The model under review builds one solid part; all positions refer to its coordinate system, in mm. Face numbers are marked on the shaded views. Round coordinates to 2 decimals unless told otherwise and drop trailing zeros. Order: outer loops, then holes, each group sorted by start corner. A loop starts at its lowest first (then second) coordinate and runs counter-clockwise, first axis right, second up. Notation, with made-up numbers: M 79.5,51 L 110.5,51 A9 cw 110.5,64 Z; hole C -25.5,-30 d9. An arc over 180 degrees is marked long. Answer as a JSON object with one key per item and string values. Group by question number.
1. Add section D-D on y = 40. State the section outline as (x, z) points, and give its area (4 significant figures).
2. To check wall thickness, follow probe 1 along X at (y, z) = (7.5, 1.4); probe 2 along X at (y, z) = (49.5, 0.75); probe 3 along Y at (x, z) = (-31, 3.5). State the ranges of each line that lie inside material, in increasing order. Write a range as [from, to].
3. Add section A-A on y = 61. State the section outline as (x, z) points, and give its area (3 significant figures).
4. Add section C-C on z = 1.65. Give the number of separate pieces and of enclosed holes in the cut face, and give its area (3 significant figures).
5. Clearance check with a flat-ended pin moving along its axis: P1, Ø1.5, axis at x = -38.5, y = 20.5, coming from the -Z side. State where the tip first meets the part, or that it passes through.
6. Add section B-B on x = -39.5. State the section outline as (y, z) points, and give its area (3 significant figures).
7. Mouldability with a two-part tool opening along Y and no side actions: class the marked faces 1, 2 and 3 as released by +Y, released by -Y, zero draft, split by the parting line, or undercut.
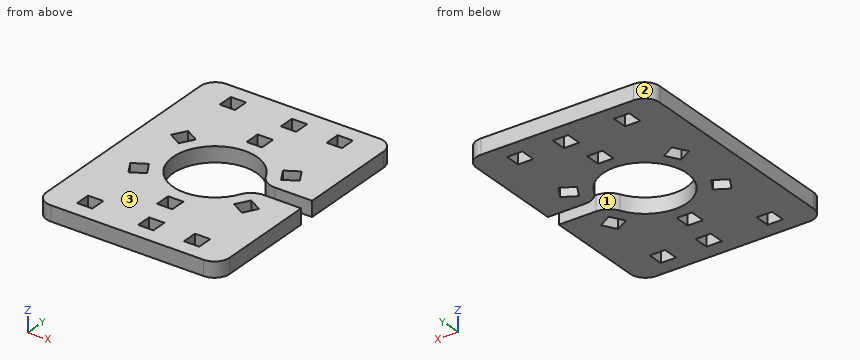
```python
from build123d import *

# Parameters (mm, degrees)
ESQUISSE1_W        = 5
ESQUISSE1_H        = 5
BOSS_EXTRU_1_DEPTH = 5


with BuildPart() as part:
    # Esquisse1 → Boss.-Extru.1 (new body)
    with BuildSketch(Plane.XY):
        with BuildLine():
            Line((-55, 80), (-5, 80))
            ThreePointArc((-5, 80), (-1.464466094, 78.535533906), (0, 75))
            Line((0, 75), (0, 42.5))
            Line((0, 42.5), (-12.172703514, 42.5))
            ThreePointArc((-12.172703514, 42.5), (-15.374759815, 43.42586604), (-17.588591054, 45.917721519))
            ThreePointArc((-17.588591054, 45.917721519), (-43.75, 40), (-17.588591054, 34.082278481))
            ThreePointArc((-17.588591054, 34.082278481), (-15.374759815, 36.57413396), (-12.172703514, 37.5))
            Line((-12.172703514, 37.5), (0, 37.5))
            Line((0, 37.5), (0, 5))
            ThreePointArc((0, 5), (-1.464466094, 1.464466094), (-5, 0))
            Line((-5, 0), (-55, 0))
            ThreePointArc((-55, 0), (-58.535533906, 1.464466094), (-60, 5))
            Line((-60, 5), (-60, 75))
            ThreePointArc((-60, 75), (-58.535533906, 78.535533906), (-55, 80))
        make_face()
        with Locations((-12.5, 72.5)):
            Rectangle(ESQUISSE1_W, ESQUISSE1_H, mode=Mode.SUBTRACT)
        with Locations((-47.5, 7.5)):
            Rectangle(ESQUISSE1_W, ESQUISSE1_H, mode=Mode.SUBTRACT)
        with Locations((-27.5, 7.5)):
            Rectangle(ESQUISSE1_W, ESQUISSE1_H, mode=Mode.SUBTRACT)
        with Locations((-12.5, 7.5)):
            Rectangle(ESQUISSE1_W, ESQUISSE1_H, mode=Mode.SUBTRACT)
        with Locations((-27.5, 72.5)):
            Rectangle(ESQUISSE1_W, ESQUISSE1_H, mode=Mode.SUBTRACT)
        with Locations((-47.5, 72.5)):
            Rectangle(ESQUISSE1_W, ESQUISSE1_H, mode=Mode.SUBTRACT)
        with Locations((-30, 60.4)):
            Rectangle(ESQUISSE1_W, ESQUISSE1_H, mode=Mode.SUBTRACT)
        Polygon((-11.418018253, 53.615063509), (-8.918018253, 49.284936491), (-13.248145272, 46.784936491), (-15.748145272, 51.115063509), align=None, mode=Mode.SUBTRACT)
        Polygon((-8.918018253, 30.715063509), (-11.418018253, 26.384936491), (-15.748145272, 28.884936491), (-13.248145272, 33.215063509), align=None, mode=Mode.SUBTRACT)
        with Locations((-30, 19.6)):
            Rectangle(ESQUISSE1_W, ESQUISSE1_H, mode=Mode.SUBTRACT)
        Polygon((-48.581981747, 26.384936491), (-51.081981747, 30.715063509), (-46.751854728, 33.215063509), (-44.251854728, 28.884936491), align=None, mode=Mode.SUBTRACT)
        Polygon((-51.081981747, 49.284936491), (-48.581981747, 53.615063509), (-44.251854728, 51.115063509), (-46.751854728, 46.784936491), align=None, mode=Mode.SUBTRACT)
    extrude(amount=BOSS_EXTRU_1_DEPTH)


solid = part.part
```
Recorded:
{
 "1": {"outline": "M -60,0 L -43.75,0 L -43.75,5 L -60,5 Z", "area": "81.25 mm²"},
 "2": {"probe 1": "x = [-60, -50], [-45, -30], [-25, -15], [-10, 0]", "probe 2": "x = [-60, -50.96], [-45.18, -39.94], [-20.06, -14.82], [-9.04, 0]", "probe 3": "y = [0, 17.1], [22.1, 26.29], [53.71, 57.9], [62.9, 80]"},
 "3": {"outline": "M -60,0 L -32.5,0 L -32.5,5 L -60,5 Z; M -27.5,0 L 0,0 L 0,5 L -27.5,5 Z", "area": "275 mm²"},
 "4": {"separate pieces": "1", "enclosed holes": "12", "area": "3,800 mm²"},
 "5": {"P1": "stops at z = 0"},
 "6": {"outline": "M 0,0 L 30.06,0 L 30.06,5 L 0,5 Z; M 49.94,0 L 80,0 L 80,5 L 49.94,5 Z", "area": "301 mm²"},
 "7": {"face 1": "undercut", "face 2": "released by +Y", "face 3": "zero draft"}
}
